```python
from build123d import *

# Parameters (mm, degrees)
F0_W     = 101.6
F0_H     = 76.2
F1_DEPTH = 25.4
F2_R     = 6.35
F3_DEPTH = 25.4
F4_W     = 25.4
F4_H     = 50.8
F6_W     = 16.163637
F6_H     = 12.7
F8_SIZE  = 5.08
F9_R     = 5.08


with BuildPart() as f1:
    # F0 (on Top) → F1 (new body)
    with BuildSketch(Plane.XY):
        Rectangle(F0_W, F0_H)
    extrude(amount=F1_DEPTH)

    # F2 (on face) → F3 (cut)
    with BuildSketch(Plane.XY.offset(25.4)):
        with Locations((-38.1, 25.4)):
            Circle(F2_R)
        with Locations((38.1, 25.4)):
            Circle(F2_R)
        with Locations((38.1, -25.4)):
            Circle(F2_R)
        with Locations((-38.1, -25.4)):
            Circle(F2_R)
    extrude(amount=-F3_DEPTH, mode=Mode.SUBTRACT)

    # F4 (on Front) → F5 (revolve)
    with BuildSketch(Plane.XZ):
        with Locations((-12.7, 50.8)):
            Rectangle(F4_W, F4_H)
    revolve(axis=Axis((0, 0, 50.8), (0, 0, 1)))

    # F6 (on Front) → F7 (revolve, cut)
    with BuildSketch(Plane.XZ):
        with Locations((-30.018182, 53.93349)):
            Rectangle(F6_W, F6_H)
    revolve(axis=Axis((0, 0, 76.2), (0, 0, -1)), mode=Mode.SUBTRACT)

    # F8
    f8_edges = [f1.edges().sort_by_distance(p)[0] for p in [
        (0, -38.1, 25.4),
        (-50.8, 0, 25.4),
        (0, 38.1, 25.4),
        (50.8, 0, 25.4),
    ]]
    chamfer(f8_edges, length=F8_SIZE)

    # F9
    f9_edges = [f1.edges().sort_by_distance(p)[0] for p in [
        (25.4, 0, 25.4),
        (25.4, 0, 76.2),
    ]]
    fillet(f9_edges, radius=F9_R)


solid = f1.part
```
Can you work these out from the model? Positions are in its coordinate system, mm. A direction names the side the tool comes from. Coordinates: 2 decimals unless noted, no trailing zeros. Loops run counter-clockwise (first coordinate to the right, second up) from the corner with the lowest first, then second, coordinate; pieces in that order, holes last. Notation, with made-up numbers: (-0.75, -2.75) - (3.25, -2.75) arc R21 ccw to (3.25, 7.25) - close; hole circle Ø5 at (-27, 69). An arc over 180 degrees is marked (long way). Answer as CSV lines item,"result". Start each with the question number.
1) Suppose I cut it at C-C (y = 0). Please give me the cut outline in (x, z).
2) Thinking about a two-plate mould opening in Y: for faces 1 (the cylindrical face through (-32.234, 22.968, 12.878)), 2 (the flat face through (50.8, -1, 10)), 3 (the cylindrical face through (31.756, 25.679, 12.878)), 4 (the flat face through (-1, 38.1, 10)), which applies, pulls with the +Y half, pulls with the -Y half, needs draft (parallel to the pull), parting line crosses it, or undercut?
3) I need wall thicknesses on line 1 (Y direction, x = 38.1, z = 15); line 2 (X direction, y = 24.5, z = 25); line 3 (Y direction, x = -35.5, z = 9). Which ranges of each line are inside material? Lowest first, please. Write a range as from..to.
4) Suppose I cut it at A-A (x = -38.1). Please give me the cut outline in (y, z).
5) For pin 1 (14.5 mm diameter, centred on x = -38.1, y = -25.4, fed in from +Z); pin 2 (1.5 mm diameter, centred on y = -22.5, z = 33, fed in from +X), each with a flat end and sliding along its axis, tell me the tip position at first contact or that it passes through.
6) Which directions (+Z, -Z, +X, -X, +Y, -Y) give clear straight access to the entire face, cutting with the end or side of a thin tool? Please do faces 5 (the flat face through (-1, 1, 0)), 6 (the cylindrical face through (4.755, -21.415, 54.022)), 7 (the flat face through (-21, 22.5, 25.4)).
7) Suppose I cut it at B-B (x = 0). Please give me the cut outline in (y, z).
8) Suppose I cut it at D-D (z = 51.5). Please give me the cut outline in (x, y).
Check result:
1,outline,"(-50.8, 0) - (50.8, 0) - (50.8, 20.32) - (45.72, 25.4) - (30.48, 25.4) arc R5.08 cw to (25.4, 30.48) - (25.4, 47.58) - (21.94, 47.58) - (21.94, 60.28) - (25.4, 60.28) - (25.4, 71.12) arc R5.08 ccw to (20.32, 76.2) - (-20.32, 76.2) arc R5.08 ccw to (-25.4, 71.12) - (-25.4, 60.28) - (-21.94, 60.28) - (-21.94, 47.58) - (-25.4, 47.58) - (-25.4, 30.48) arc R5.08 cw to (-30.48, 25.4) - (-45.72, 25.4) - (-50.8, 20.32) - close"
2,face 1,"undercut"
2,face 2,"needs draft"
2,face 3,"undercut"
2,face 4,"pulls with the +Y half"
3,line 1,"y = -38.1..-31.75, -19.05..19.05, 31.75..38.1"
3,line 2,"x = -46.12..-44.39, -31.81..31.81, 44.39..46.12"
3,line 3,"y = -38.1..-31.19, -19.61..19.61, 31.19..38.1"
4,outline,"(-38.1, 0) - (-31.75, 0) - (-31.75, 25.4) - (-33.02, 25.4) - (-38.1, 20.32) - close; (-19.05, 0) - (19.05, 0) - (19.05, 25.4) - (-19.05, 25.4) - close; (31.75, 0) - (38.1, 0) - (38.1, 20.32) - (33.02, 25.4) - (31.75, 25.4) - close"
5,pin 1,"stops at z = 25.4"
5,pin 2,"stops at x = 13.12"
6,face 5,"-Z, +X, -X, +Y, -Y"
6,face 6,"none"
6,face 7,"+Z"
7,outline,"(-38.1, 0) - (38.1, 0) - (38.1, 20.32) - (33.02, 25.4) - (30.48, 25.4) arc R5.08 cw to (25.4, 30.48) - (25.4, 47.58) - (21.94, 47.58) - (21.94, 60.28) - (25.4, 60.28) - (25.4, 71.12) arc R5.08 ccw to (20.32, 76.2) - (-20.32, 76.2) arc R5.08 ccw to (-25.4, 71.12) - (-25.4, 60.28) - (-21.94, 60.28) - (-21.94, 47.58) - (-25.4, 47.58) - (-25.4, 30.48) arc R5.08 cw to (-30.48, 25.4) - (-33.02, 25.4) - (-38.1, 20.32) - close"
8,outline,"circle Ø43.87 at (0, 0)"
